```python
from build123d import *

# Parameters (mm, degrees)
SKETCH1_W           = 33.7
SKETCH1_H           = 12
BOSS_EXTRUDE1_DEPTH = 2.5
SKETCH2_W           = 33.7
SKETCH2_H           = 4.5
BOSS_EXTRUDE2_DEPTH = 17.5
SKETCH3_W           = 13
SKETCH3_H           = 23.5
CUT_EXTRUDE1_DEPTH  = 258.235074474
SKETCH4_W           = 2.85
SKETCH4_H           = 12
BOSS_EXTRUDE3_DEPTH = 23.5
FILLET1_R           = 6
SKETCH5_R           = 3.5
CUT_EXTRUDE2_DEPTH  = 4
SKETCH6_R           = 3
CUT_EXTRUDE3_DEPTH  = 4
SKETCH7_W           = 3.5
SKETCH7_H           = 12
BOSS_EXTRUDE4_DEPTH = 11.77
FILLET2_R           = 1
SKETCH8_R           = 0.8
CUT_EXTRUDE4_DEPTH  = 2


with BuildPart() as part:
    # Sketch1 → Boss-Extrude1 (new body)
    with BuildSketch(Plane(origin=(0, 0, 0), x_dir=(0, 0, -1), z_dir=(1, 0, 0))):
        with Locations((-239.496705732, 20.068965517)):
            Rectangle(SKETCH1_W, SKETCH1_H)
    extrude(amount=BOSS_EXTRUDE1_DEPTH)

    # Sketch2 → Boss-Extrude2 (add)
    with BuildSketch(Plane(origin=(2.5, 0, 0), x_dir=(0, 0, -1), z_dir=(1, 0, 0))):
        with Locations((-239.496705732, 16.318965517)):
            Rectangle(SKETCH2_W, SKETCH2_H)
    extrude(amount=BOSS_EXTRUDE2_DEPTH)

    # Sketch3 → Cut-Extrude1 (cut, through all)
    with BuildSketch(Plane(origin=(0, 18.568965517, 0), x_dir=(1, 0, 0), z_dir=(0, 1, 0))):
        with Locations((10, -239.496705732)):
            Rectangle(SKETCH3_W, SKETCH3_H)
    extrude(amount=-CUT_EXTRUDE1_DEPTH, mode=Mode.SUBTRACT)

    # Sketch4 → Boss-Extrude3 (add)
    with BuildSketch(Plane.ZY):
        with Locations((224.071705732, 20.068965517)):
            Rectangle(SKETCH4_W, SKETCH4_H)
        with Locations((254.921705732, 20.068965517)):
            Rectangle(SKETCH4_W, SKETCH4_H)
    extrude(amount=BOSS_EXTRUDE3_DEPTH)

    # Fillet1
    fillet1_edges = [part.edges().sort_by_distance(p)[0] for p in [
        (-23.5, 14.068965517, 224.071705732),
        (-23.5, 26.068965517, 224.071705732),
        (-23.5, 14.068965517, 254.921705732),
        (-23.5, 26.068965517, 254.921705732),
    ]]
    fillet(fillet1_edges, radius=FILLET1_R - 0.0001)  # a hair under: the kernel refuses the full size

    # Sketch5 → Cut-Extrude2 (cut)
    with BuildSketch(Plane.XY.offset(256.346705732)):
        with Locations((-17.5, 20.068965517)):
            Circle(SKETCH5_R)
    extrude(amount=-CUT_EXTRUDE2_DEPTH, mode=Mode.SUBTRACT)

    # Sketch6 → Cut-Extrude3 (cut)
    with BuildSketch(Plane.XY.offset(225.496705732)):
        with Locations((-17.5, 20.068965517)):
            Circle(SKETCH6_R)
    extrude(amount=-CUT_EXTRUDE3_DEPTH, mode=Mode.SUBTRACT)

    # Sketch7 → Boss-Extrude4 (add)
    with BuildSketch(Plane(origin=(0, 18.568965517, 0), x_dir=(1, 0, 0), z_dir=(0, 1, 0))):
        with Locations((1.75, -234.246705732)):
            Rectangle(SKETCH7_W, SKETCH7_H)
    extrude(amount=BOSS_EXTRUDE4_DEPTH)

    # Fillet2
    fillet2_edges = [part.edges().sort_by_distance(p)[0] for p in [
        (2.5, 22.318965517, 222.646705732),
        (11.25, 18.568965517, 256.346705732),
        (11.25, 18.568965517, 222.646705732),
        (20, 16.318965517, 256.346705732),
        (20, 14.068965517, 239.496705732),
        (20, 16.318965517, 222.646705732),
        (20, 18.568965517, 239.496705732),
        (2.5, 22.318965517, 256.346705732),
        (-21.742669976, 24.311635494, 222.646705732),
        (-21.742669976, 15.826295541, 222.646705732),
        (-21.742669976, 24.311635494, 256.346705732),
        (-21.742669976, 15.826295541, 256.346705732),
        (-7.50005, 26.068965517, 256.346705732),
        (-7.50005, 26.068965517, 222.646705732),
        (1.24995, 14.068965517, 222.646705732),
        (1.24995, 14.068965517, 256.346705732),
    ]]
    fillet(fillet2_edges, radius=FILLET2_R)

    # Sketch8 → Cut-Extrude4 (cut)
    with BuildSketch(Plane(origin=(0, 30.338965517, 0), x_dir=(1, 0, 0), z_dir=(0, 1, 0))):
        with Locations(Location((1.75, -231.246705732, 0), (0, 0, 270))):
            Circle(SKETCH8_R)
        with Locations(Location((1.75, -237.246705732, 0), (0, 0, 270))):
            Circle(SKETCH8_R)
    extrude(amount=-CUT_EXTRUDE4_DEPTH, mode=Mode.SUBTRACT)


solid = part.part
```
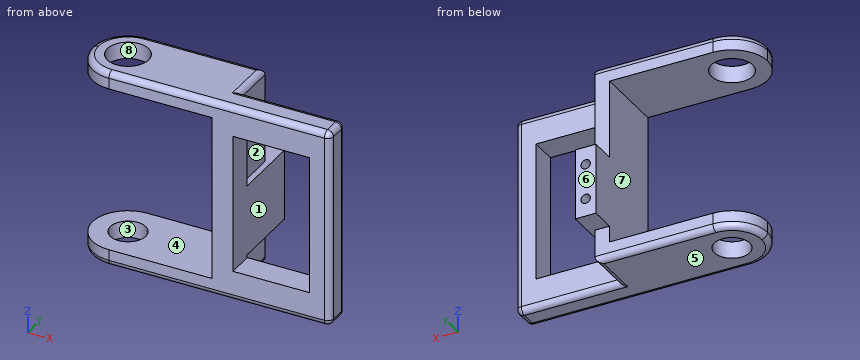
The listing builds one solid part. Answer for the finished solid, in the listing's coordinates (mm). Face numbers are marked on the shaded views. A direction names the side the tool comes from. Give positions to 0.01 mm unless a question says otherwise; leave off trailing zeros. Order: outer loops, then holes, each group sorted by start corner. A loop starts at its lowest first (then second) coordinate and runs counter-clockwise, first axis right, second up. Notation, with made-up numbers: (32, 57) -> (57, 57) arc R20 cw to (57, 80) -> close; hole circle Ø10 at (-2, -19). An arc over 180 degrees is marked (long way). Write each question's results on one line, items separated by ' | '.
Q1. The part is cut by section A-A, the plane x = -0.5. Give the vertices of the cut face in (y, z), and give its area (3 significant figures).
Checked values:
outline: (14.07, 223.65) arc R1 ccw to (15.07, 222.65) -> (25.07, 222.65) arc R1 ccw to (26.07, 223.65) -> (26.07, 225.5) -> (14.07, 225.5) -> close; (14.07, 253.5) -> (26.07, 253.5) -> (26.07, 255.35) arc R1 ccw to (25.07, 256.35) -> (15.07, 256.35) arc R1 ccw to (14.07, 255.35) -> close | area: 67.5 mm^2
Q2. The part is cut by section C-C, the plane x = -17. Give the vertices of the cut face in (y, z), and give its area (3 significant figures).
Checked values:
outline: (14.07, 223.65) arc R1 ccw to (15.07, 222.65) -> (17.11, 222.65) -> (17.11, 225.5) -> (14.07, 225.5) -> close; (14.07, 253.5) -> (16.6, 253.5) -> (16.6, 256.35) -> (15.07, 256.35) arc R1 ccw to (14.07, 255.35) -> close; (23.03, 222.65) -> (25.07, 222.65) arc R1 ccw to (26.07, 223.65) -> (26.07, 225.5) -> (23.03, 225.5) -> close; (23.53, 253.5) -> (26.07, 253.5) -> (26.07, 255.35) arc R1 ccw to (25.07, 256.35) -> (23.53, 256.35) -> close | area: 30.9 mm^2
Q3. Which of the six approach directions +Z, -Z, +X, -X, +Y, -Y give full straight-line access (tool end or side, diameter ignored) to the marked faces 1, 2, 3, 4 and 5?
Checked values:
face 1: +Y, -Y | face 2: +Z, +X, +Y | face 3: +Z, -Z | face 4: -X, +Y, -Y | face 5: -Z, +X, -X, +Y, -Y
Q4. The part is cut by section B-B, the plane z = 242.5. Give the vertices of the cut face in (x, y).
Checked values:
outline: (0, 14.07) -> (3.5, 14.07) -> (3.5, 18.57) -> (2.5, 18.57) -> (2.5, 26.07) -> (0, 26.07) -> close; (16.5, 14.07) -> (19, 14.07) arc R1 ccw to (20, 15.07) -> (20, 17.57) arc R1 ccw to (19, 18.57) -> (16.5, 18.57) -> close
Q5. The part is cut by section D-D, the plane y = 21.5. State how many separate pieces and enclosed holes the cut face has, and give its area (3 significant figures).
Checked values:
separate pieces: 3 | enclosed holes: 0 | area: 195 mm^2
Q6. Each of these flat-tipped pins is pushed along its axis until it touches: P1, Ø7.5, axis at x = -12, z = 248.5, coming from the +Y side; P2, Ø2, axis at y = 20, z = 239.5, coming from the -X side; P3, Ø2, axis at y = 21.5, z = 250, coming from the +X side; P4, Ø1.5, axis at y = 23, z = 238.5, coming from the +X side. Where does it stop, or does it pass through?
Checked values:
P1: passes through | P2: stops at x = 0 | P3: stops at x = 2.5 | P4: stops at x = 3.5
Q7. Determine the mould class of the marked faces 6, 7 and 8 for opening direction Y: pulls with the +Y half, pulls with the -Y half, needs draft (parallel to the pull), parting line crosses it, or undercut.
Checked values:
face 6: pulls with the +Y half | face 7: needs draft | face 8: undercut
Q8. Straight lines are drawn through the part: probe 1 along Z at (x, y) = (-19, 23.5); probe 2 along Y at (x, z) = (3, 250.5); probe 3 along Y at (x, z) = (-3.5, 254). For each, find the intervals that lie inside material, in ascending order. Write a range as from..to.
Checked values:
probe 1: z = 222.65..225.5, 253.5..256.35 | probe 2: y = 14.07..18.57 | probe 3: y = 14.07..26.07
